The listing builds one solid part. Answer for the finished solid, in the listing's coordinates (mm). Face numbers are marked on the shaded views. Coordinates: 2 decimals unless noted, no trailing zeros. Order: outer loops, then holes, each group sorted by start corner. A loop starts at its lowest first (then second) coordinate and runs counter-clockwise, first axis right, second up. Notation, with made-up numbers: (8, 58) - (65, 58) arc R13 cw to (65, 67) - close; hole circle Ø5 at (-4, -7.5). An arc over 180 degrees is marked (long way). Use one line per item in the form item = value. Start each with the question number.
Item 1: Each of these flat-tipped pins is pushed along its axis until it touches: pin 1 Ø4 at (x, z) = (40, -13) entering from -Y; pin 2 Ø12 at (x, y) = (-4, 30) entering from +Z; pin 3 Ø8 at (y, z) = (-19.5, -12.5) entering from +X. Where does it stop, or does it pass through?
Item 2: Consider line 1 along Y through (x, z) = (0, 53); line 2 along Y through (x, z) = (-11, 24); line 3 along X through (y, z) = (-18, -46). Determine where each line is inside the solid, lowest interval first. Write a range as [from, to].
Item 3: The mould has two halves that part along Y. Classify the marked faces 1 and 2: released by +Y, released by -Y, zero draft, split by the parting line, or undercut.
Item 4: Section A-A, the plane z = -7 is taken. Write down the section's boundary in (x, y), and give its area (3 significant figures).
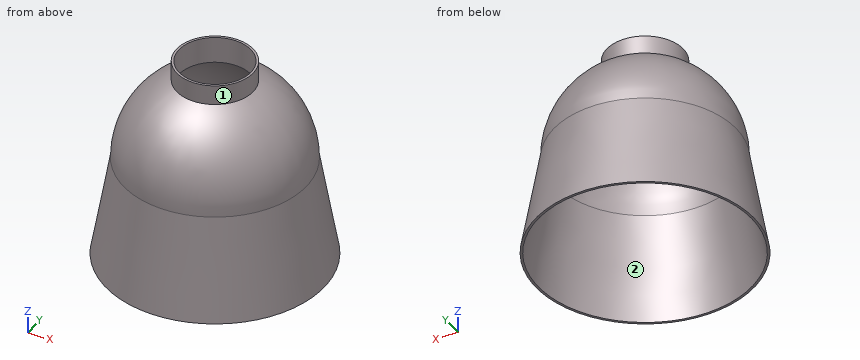
from build123d import *

# Parameters (mm, degrees)
F2_R     = 21.2725
F2_R_2   = 20
F3_DEPTH = 57.15
F4_DEPTH = 57.151
F5_DEPTH = 42.545


with BuildPart() as f1:
    # F0 (on Front) → F1 (revolve)
    with BuildSketch(Plane.XZ):
        with BuildLine():
            Line((0, 49.53), (0, 50.8))
            ThreePointArc((0, 50.8), (-35.921024, 35.921024), (-50.8, 0))
            Line((-50.8, 0), (-49.53, 0))
            ThreePointArc((-49.53, 0), (-35.022999, 35.022999), (0, 49.53))
        make_face()
        Polygon((-49.53, 0), (-50.8, 0), (-60.723993, -56.281763), (-59.453993, -56.281763), align=None)
    revolve(axis=Axis((0, 0, -2.740882), (0, 0, -1)))

    # F2 (on Top) → F3 (join)
    with BuildSketch(Plane.XY):
        Circle(F2_R)
        Circle(F2_R_2, mode=Mode.SUBTRACT)
    extrude(amount=F3_DEPTH)

    # F2 (on Top) → F4 (cut, through all)
    with BuildSketch(Plane.XY):
        Circle(F2_R_2)
    extrude(amount=F4_DEPTH, mode=Mode.SUBTRACT)

    # F2 (on Top) → F5 (cut)
    with BuildSketch(Plane.XY):
        Circle(F2_R_2)
        Circle(F2_R)
        Circle(F2_R_2, mode=Mode.SUBTRACT)
    extrude(amount=F5_DEPTH, mode=Mode.SUBTRACT)


solid = f1.part
Response:
q1.pin_1 = -37.14
q1.pin_2 = 44.63
q1.pin_3 = 50.89
q2.line_1 = [-21.27, -20], [20, 21.27]
q2.line_2 = [-43.4, -41.91], [41.91, 43.4]
q2.line_3 = [-56.09, -54.76], [54.76, 56.09]
q3.face_1 = split by the parting line
q3.face_2 = undercut
q4.outline = circle Ø104.07 at (0, 0); hole circle Ø101.53 at (0, 0)
q4.area = 410 mm2
